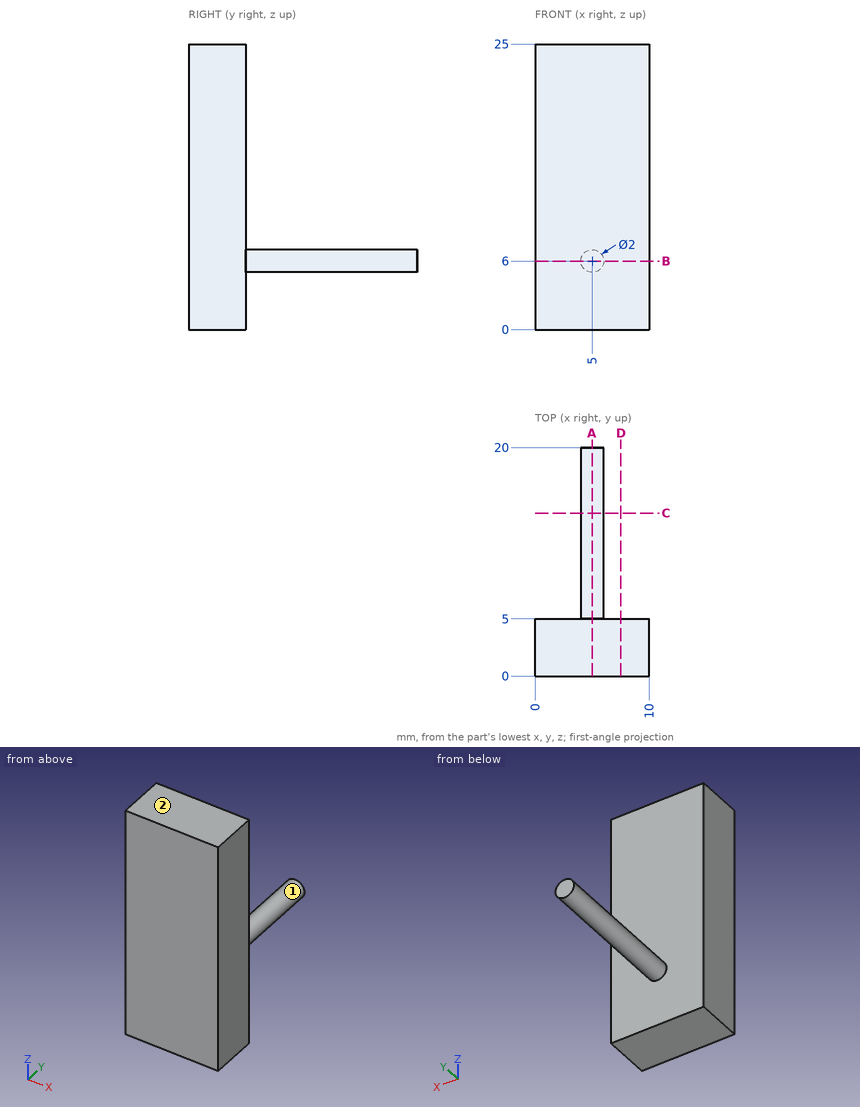
Geometry: see drawing. Coordinates: mm, zero at the bounding-box minimum. A direction names the side the tool comes from. Give positions to 0.01 mm unless a question says otherwise; leave off trailing zeros. Order: outer loops, then holes, each group sorted by start corner. A loop starts at its lowest first (then second) coordinate and runs counter-clockwise, first axis right, second up. Notation, with made-up numbers: (86.5, 53) - (123.5, 53) arc R10 ccw to (123.5, 69) - close; hole circle Ø5 at (-33.5, 32). An arc over 180 degrees is marked (long way). Use a Markdown table: item, result.
(1) Line query: line 1 (Y direction, x = 1.5, z = 17); line 2 (Z direction, x = 5.25, y = 13.5). Output: solid intervals per line, ascending. Write a range as from..to.
Computed values:
| item | result |
|---|---|
| line 1 | y = 0..5 |
| line 2 | z = 5.03..6.97 |
(2) Section query B-B (z = 6). Output: boundary loops of the cut face in (x, y), then the cut area to 3 significant figures.
Computed values:
| item | result |
|---|---|
| outline | (0, 0) - (10, 0) - (10, 5) - (6, 5) - (6, 20) - (4, 20) - (4, 5) - (0, 5) - close |
| area | 80.0 mm2 |
(3) Section query C-C (y = 14.25). Output: boundary loops of the cut face in (x, z).
Computed values:
| item | result |
|---|---|
| outline | circle Ø2 at (5, 6) |
(4) Section query D-D (x = 7.5). Output: boundary loops of the cut face in (y, z).
Computed values:
| item | result |
|---|---|
| outline | (0, 0) - (5, 0) - (5, 25) - (0, 25) - close |
(5) Pin query (flat end, axial travel): pin 1 (2 mm diameter, centred on x = 1.5, y = 13, fed in from -Z); pin 2 (5 mm diameter, centred on x = 4.5, y = 16.5, fed in from -Z). Return the tip coordinate at first contact, or that it passes through.
Computed values:
| item | result |
|---|---|
| pin 1 | passes through |
| pin 2 | stops at z = 5 |
(6) Access query for the marked faces 1 and 2. Directions: +Z, -Z, +X, -X, +Y, -Y. A direction counts if a zero-diameter tool reaches every point of the face in a straight line with its end or side. Return the directions, or none.
Computed values:
| item | result |
|---|---|
| face 1 | +Y |
| face 2 | +Z, +X, -X, +Y, -Y |
(7) Section query A-A (x = 5). Output: boundary loops of the cut face in (y, z), then the cut area to 3 significant figures.
Computed values:
| item | result |
|---|---|
| outline | (0, 0) - (5, 0) - (5, 5) - (20, 5) - (20, 7) - (5, 7) - (5, 25) - (0, 25) - close |
| area | 155 mm2 |
